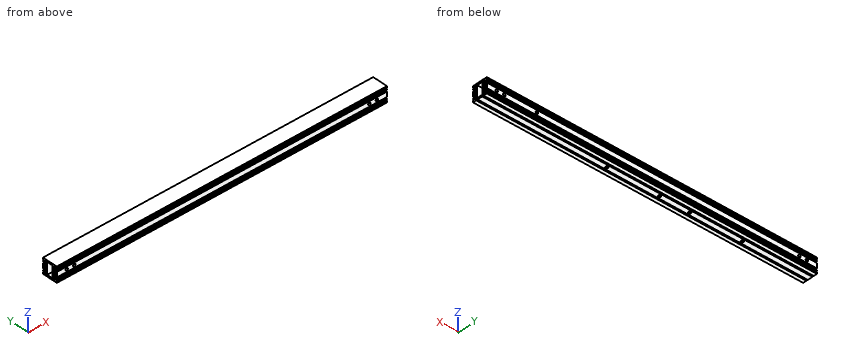
from build123d import *

# Parameters (mm, degrees)
SKETCH_1_W             = 23.5
SKETCH_1_H             = 12
EXTRUDE_1_DEPTH        = 329
HOLE_WIZARD_M6_1_D     = 5
HOLE_WIZARD_M6_1_DEPTH = 19
HOLE_WIZARD_M6_1_TIP   = 1.502151548
HOLE_WIZARD_M6_2_D     = 5
HOLE_WIZARD_M6_2_DEPTH = 19
HOLE_WIZARD_M6_2_TIP   = 1.502151548
HOLE_WIZARD_M6_3_D     = 5
HOLE_WIZARD_M6_3_DEPTH = 19
HOLE_WIZARD_M6_3_TIP   = 1.502151548


with BuildPart() as part:
    # 草图1 → 凸台-拉伸1 (new, symmetric)
    with BuildSketch(Plane(origin=(0, 0, 0), x_dir=(0, 0, -1), z_dir=(1, 0, 0))):
        Polygon((-15, 15), (-11.5, 15), (-11.5, 13.5), (-11, 13.5), (-11, 12), (-9.5, 12), (-9.5, 15), (-8, 15), (-8, 12.5), (-5, 12.5), (-5, 15), (5, 15), (5, 12.5), (8, 12.5), (8, 15), (9.5, 15), (9.5, 12), (11, 12), (11, 13.5), (11.5, 13.5), (11.5, 15), (15, 15), (15, 8), (12.5, 8), (12.5, 5), (15, 5), (15, -5), (12.5, -5), (12.5, -8), (15, -8), (15, -15), (11.5, -15), (11.5, -13.5), (11, -13.5), (11, -12), (9.5, -12), (9.5, -15), (8, -15), (8, -12.5), (5, -12.5), (5, -15), (-5, -15), (-5, -12.5), (-8, -12.5), (-8, -15), (-9.5, -15), (-9.5, -12), (-11, -12), (-11, -13.5), (-11.5, -13.5), (-11.5, -15), (-15, -15), align=None)
        with BuildLine():
            Line((12, -10.5), (12, -8.5))
            ThreePointArc((12, -8.5), (11.853553391, -8.146446609), (11.5, -8))
            Line((11.5, -8), (-11.5, -8))
            ThreePointArc((-11.5, -8), (-11.853553391, -8.146446609), (-12, -8.5))
            Line((-12, -8.5), (-12, -10.5))
            ThreePointArc((-12, -10.5), (-11.853553391, -10.853553391), (-11.5, -11))
            Line((-11.5, -11), (11.5, -11))
            ThreePointArc((11.5, -11), (11.853553391, -10.853553391), (12, -10.5))
        make_face(mode=Mode.SUBTRACT)
        with BuildLine():
            Line((-11.5, 11), (11.5, 11))
            ThreePointArc((11.5, 11), (11.853553391, 10.853553391), (12, 10.5))
            Line((12, 10.5), (12, 8.5))
            ThreePointArc((12, 8.5), (11.853553391, 8.146446609), (11.5, 8))
            Line((11.5, 8), (-11.5, 8))
            ThreePointArc((-11.5, 8), (-11.853553391, 8.146446609), (-12, 8.5))
            Line((-12, 8.5), (-12, 10.5))
            ThreePointArc((-12, 10.5), (-11.853553391, 10.853553391), (-11.5, 11))
        make_face(mode=Mode.SUBTRACT)
        Rectangle(SKETCH_1_W, SKETCH_1_H, mode=Mode.SUBTRACT)
    extrude(amount=EXTRUDE_1_DEPTH, both=True)

    # M6 螺纹孔1
    with Locations(Plane(origin=(0, 15, 0), x_dir=(1, 0, 0), z_dir=(0, 1, 0))):
        with Locations((-309, 0), (-294, 0), (294, 0), (309, 0), (229, 0)):
            Hole(HOLE_WIZARD_M6_1_D / 2, depth=HOLE_WIZARD_M6_1_DEPTH)
            with Locations((0, 0, -(HOLE_WIZARD_M6_1_DEPTH + HOLE_WIZARD_M6_1_TIP / 2))):  # 118° drill point
                Cone(0, HOLE_WIZARD_M6_1_D / 2, HOLE_WIZARD_M6_1_TIP, mode=Mode.SUBTRACT)

    # M6 螺纹孔2
    with Locations(Plane(origin=(0, -15, 0), x_dir=(-1, 0, 0), z_dir=(0, -1, 0))):
        with Locations((-309, 0), (-294, 0), (309, 0), (294, 0)):
            Hole(HOLE_WIZARD_M6_2_D / 2, depth=HOLE_WIZARD_M6_2_DEPTH)
            with Locations((0, 0, -(HOLE_WIZARD_M6_2_DEPTH + HOLE_WIZARD_M6_2_TIP / 2))):  # 118° drill point
                Cone(0, HOLE_WIZARD_M6_2_D / 2, HOLE_WIZARD_M6_2_TIP, mode=Mode.SUBTRACT)

    # M6 螺纹孔3
    with Locations(Plane(origin=(0, 0, -15), x_dir=(-1, 0, 0), z_dir=(0, 0, -1))):
        with Locations((194, 0), (89, 0), (29, 0), (-76, 0)):
            Hole(HOLE_WIZARD_M6_3_D / 2, depth=HOLE_WIZARD_M6_3_DEPTH)
            with Locations((0, 0, -(HOLE_WIZARD_M6_3_DEPTH + HOLE_WIZARD_M6_3_TIP / 2))):  # 118° drill point
                Cone(0, HOLE_WIZARD_M6_3_D / 2, HOLE_WIZARD_M6_3_TIP, mode=Mode.SUBTRACT)


solid = part.part
Check sheet for the modelled part. Datum: model origin and axes. Units: mm. Give positions to 0.01 mm unless a question says otherwise; leave off trailing zeros. Write item = value, one per line.
Item 1: Gauge pin test, flat ends, axial feed: pin 1 (10 mm diameter, centred on y = -10.5, z = 6, fed in from +X); pin 2 (4.5 mm diameter, centred on x = -309, z = 0, fed in from -Y). Record the tip position at first contact, or that the pin passes through.
Output:
pin_1 = 329
pin_2 = through
Item 2: Sectioned sample at A-A on x = -109.5. Count the separate pieces of the cut face and the enclosed holes in it, and give its area (3 significant figures).
Output:
separate_pieces = 1
enclosed_holes = 3
area = 408 mm^2
Item 3: Scan lines: probe 1 along Y at (x, z) = (-139, 3.75); probe 2 along Y at (x, z) = (-250, 10.75); probe 3 along Z at (x, y) = (249.5, 13.25). Record each from-to range of solid material in increasing order. Write a range as from..to.
Output:
probe_1 = -15..-11, -8..-6, 6..8, 11..15
probe_2 = -12..-11, -8..-6, 6..8, 11..12
probe_3 = -15..-11, -9.5..-8, -5..5, 8..9.5, 11..15
